Here's how the part is built. I have some questions about the finished solid (model axes, mm). A direction names the side the tool comes from. Give positions to 0.01 mm unless a question says otherwise; leave off trailing zeros. Order: outer loops, then holes, each group sorted by start corner. A loop starts at its lowest first (then second) coordinate and runs counter-clockwise, first axis right, second up. Notation, with made-up numbers: M -34,-1.75 L -2,-1.75 A21 ccw -2,24.25 Z; hole C 51.5,4.25 d11. An arc over 180 degrees is marked long. Use one line per item in the form item = value.
from build123d import *

# Parameters (mm, degrees)
SKETCH2_R           = 10
BOSS_EXTRUDE1_DEPTH = 7
SKETCH3_R           = 10
BOSS_EXTRUDE2_DEPTH = 4
SKETCH4_R           = 7
BOSS_EXTRUDE3_DEPTH = 19
SKETCH5_R           = 3
CUT_EXTRUDE1_DEPTH  = 31
CHAMFER1_SIZE       = 0.5
CUT_EXTRUDE3_START  = 10.2
CUT_EXTRUDE3_DEPTH  = 5.8
CHAMFER2_SIZE       = 0.5


with BuildPart() as part:
    # Sketch2 → Boss-Extrude1 (new body)
    with BuildSketch(Plane.XY):
        Circle(SKETCH2_R)
    extrude(amount=BOSS_EXTRUDE1_DEPTH)

    # Sketch3 → Boss-Extrude2 (add)
    with BuildSketch(Plane.XY.offset(7)):
        with Locations((0, 5)):
            Circle(SKETCH3_R)
    extrude(amount=BOSS_EXTRUDE2_DEPTH)

    # Sketch4 → Boss-Extrude3 (add)
    with BuildSketch(Plane.XY.offset(11)):
        with Locations((0, 5)):
            Circle(SKETCH4_R)
    extrude(amount=BOSS_EXTRUDE3_DEPTH)

    # Sketch5 → Cut-Extrude1 (cut, through all)
    with BuildSketch(Plane.XY.offset(30)):
        with Locations((0, 5)):
            Circle(SKETCH5_R)
    extrude(amount=-CUT_EXTRUDE1_DEPTH, mode=Mode.SUBTRACT)

    # Chamfer1
    chamfer1_edges = [part.edges().sort_by_distance(p)[0] for p in [
        (-3, 5, 0),
        (-3, 5, 30),
    ]]
    chamfer(chamfer1_edges, length=CHAMFER1_SIZE)

    # Sketch6 → Cut-Extrude3 (cut, through all)
    with BuildSketch(Plane(origin=(0, 0, 0), x_dir=(1, 0, 0), z_dir=(0, 1, 0)).offset(CUT_EXTRUDE3_START)):
        with BuildLine():
            Line((-2.5, -16), (-2.5, -31.730265833))
            Line((-2.5, -31.730265833), (2.5, -31.730265833))
            Line((2.5, -31.730265833), (2.5, -16))
            ThreePointArc((2.5, -16), (0, -13.5), (-2.5, -16))
        make_face()
    extrude(amount=CUT_EXTRUDE3_DEPTH, mode=Mode.SUBTRACT)

    # Chamfer2
    chamfer2_edges = [part.edges().sort_by_distance(p)[0] for p in [
        (-3.968626967, -0.766281297, 30),
    ]]
    chamfer(chamfer2_edges, length=CHAMFER2_SIZE)


solid = part.part
Q1. I want a section at B-B on z = 28.5. Write out the boundary of the cut face in (x, y), then the cut area to 3 significant figures.
Found:
outline = M -2.5,10.2 L -2.5,11.54 A7 ccw long 2.5,11.54 L 2.5,10.2 Z; hole C 0,5 d6
area = 117 mm²
Q2. I want a section at A-A on x = 0. Write out the boundary of the cut face in (y, z), then the cut area to 3 significant figures.
Found:
outline = M -10,0 L 1.5,0 L 2,0.5 L 2,29.5 L 1.5,30 L -1.5,30 L -2,29.5 L -2,11 L -5,11 L -5,7 L -10,7 Z; M 8,0.5 L 8.5,0 L 10,0 L 10,7 L 15,7 L 15,11 L 12,11 L 12,13.5 L 10.2,13.5 L 10.2,30 L 8.5,30 L 8,29.5 Z
area = 276 mm²
Q3. I want a section at C-C on x = -9. Write out the boundary of the cut face in (y, z), then the cut area to 3 significant figures.
Found:
outline = M -4.36,0 L 4.36,0 L 4.36,7 L 9.36,7 L 9.36,11 L 0.64,11 L 0.64,7 L -4.36,7 Z
area = 95.9 mm²
Q4. I'm going to push flat-ended pins straight in: pin 1 Ø12 at (x, z) = (3, 3.5) entering from +Y; pin 2 Ø12 at (y, z) = (10.5, 18.5) entering from +X; pin 3 Ø1.1 at (y, z) = (11, 20.5) entering from -X; pin 4 Ø5 at (y, z) = (-4.5, 11) entering from +X. Where does each tip first touch, or does it pass through?
Found:
pin_1 = 15
pin_2 = 7
pin_3 = -4.39
pin_4 = 7.14
Q5. On a 3-axis mill with a long thin cutter (end or side, diameter ignored), from which of +Z, -Z, +X, -X, +Y, -Y can I reach the whole of each face in a straight line? I mean faces 1 (the face through (-1.302, 14.915, 8.972)), 2 (the face through (-0.1, 10.2, 7)), 3 (the face through (0.1, 10.9, 13.5)). Say none if no direction works.
Found:
face_1 = +Z
face_2 = -Z, +Y
face_3 = +Z, +Y
Q6. I want a section at D-D on y = -2.5. Write out the boundary of the cut face in (x, z).
Found:
outline = M -9.68,0 L 9.68,0 L 9.68,7 L 6.61,7 L 6.61,11 L -6.61,11 L -6.61,7 L -9.68,7 Z
Q7. I need wall thicknesses on L1, parallel to Y at x = 0, z = 15.25; L2, parallel to Z at x = -7.5, y = 2.5; L3, parallel to Y at x = -1.5, z = 3.5. Which ranges of each line are inside material? Lowest first, please.
Found:
L1 = -2 to 2, 8 to 10.2
L2 = 0 to 11
L3 = -9.89 to 2.4, 7.6 to 9.89
